```python
from build123d import *

# Parameters (mm, degrees)
SKETCH2_W           = 38.1
SKETCH2_H           = 76.2
BOSS_EXTRUDE1_DEPTH = 9.525
SKETCH3_OUTSIDE_W   = 57.246
SKETCH3_OUTSIDE_H   = 95.346
SKETCH3_OUTSIDE_W_2 = 38.1
SKETCH3_OUTSIDE_H_2 = 76.2
SKETCH3_OUTSIDE_R   = 4.318
CUT_EXTRUDE2_DEPTH  = 12.7


with BuildPart() as part:
    # Sketch2 → Boss-Extrude1 (new body)
    with BuildSketch(Plane.XY):
        Rectangle(SKETCH2_W, SKETCH2_H)
    extrude(amount=BOSS_EXTRUDE1_DEPTH)

    # Sketch3 outside → Cut-Extrude2 (cut)
    # profile 1 of 2: a face of its own
    with BuildSketch(Plane.XY.offset(9.525)):
        Rectangle(SKETCH3_OUTSIDE_W, SKETCH3_OUTSIDE_H)
        Rectangle(SKETCH3_OUTSIDE_W_2, SKETCH3_OUTSIDE_H_2, mode=Mode.SUBTRACT)
    # profile 2 of 2: a face of its own
    with BuildSketch(Plane.XY.offset(9.525)):
        Circle(SKETCH3_OUTSIDE_R)
    extrude(amount=-CUT_EXTRUDE2_DEPTH, mode=Mode.SUBTRACT)


solid = part.part
```
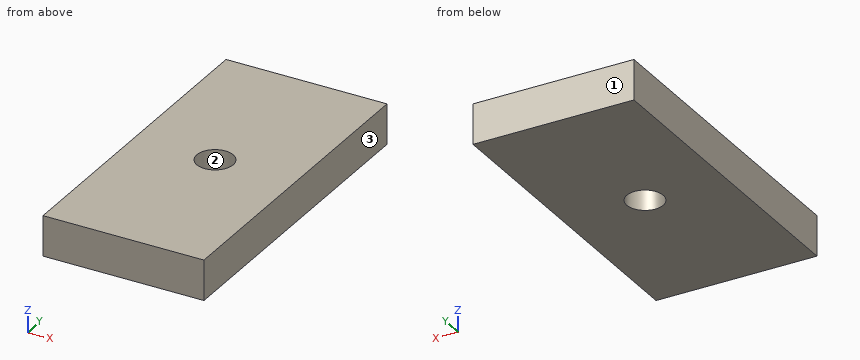
Build history of the part. All positions in model axes, mm. Face numbers are marked on the shaded views. Round coordinates to 2 decimals unless told otherwise and drop trailing zeros. Write each loop counter-clockwise with the first axis right and the second up, starting at its lowest first coordinate (ties: lowest second). Pieces come first, ordered by that corner, then holes. Notation, with made-up numbers: (39.25, 3.25) - (97.25, 3.25) arc R12 ccw to (97.25, 13.25) - close; hole circle Ø3 at (-37, -12). An arc over 180 degrees is marked (long way). Answer as CSV lines item,"result".
Q1. Pull direction Y, two halves, no side cores. Call the marked faces 1, 2 and 3: +Y half, -Y half, draft (parallel to the pull), parting line (faces both ways), or undercut.
Report:
face 1,"+Y half"
face 2,"undercut"
face 3,"draft"
Q2. Drill centre lines: probe 1 along Y at (x, z) = (0, 3.5); probe 2 along Y at (x, z) = (2, 7.75). Where is each one in solid material? Low to high. Write a range as [from, to].
Report:
probe 1,"y = [-38.1, -4.32], [4.32, 38.1]"
probe 2,"y = [-38.1, -3.83], [3.83, 38.1]"
Q3. Cut at B-B (z = 1). Write the cut outline in (x, y), and give its area (3 significant figures).
Report:
outline,"(-19.05, -38.1) - (19.05, -38.1) - (19.05, 38.1) - (-19.05, 38.1) - close; hole circle Ø8.64 at (0, 0)"
area,"2,840 mm^2"
Q4. Drop a flat-ended pin along its axis: pin 1 (5 mm diameter, centred on x = 0, y = 0, fed in from -Z). Give the stop position or say it passes through.
Report:
pin 1,"passes through"
Q5. Cut at A-A (y = 0). Write the cut outline in (x, z) (3 decimals), and give its area (3 significant figures).
Report:
outline,"(-19.05, 0) - (-4.318, 0) - (-4.318, 9.525) - (-19.05, 9.525) - close; (4.318, 0) - (19.05, 0) - (19.05, 9.525) - (4.318, 9.525) - close"
area,"281 mm^2"
Q6. Cut at C-C (x = 0). Write the cut outline in (y, z) (3 decimals).
Report:
outline,"(-38.1, 0) - (-4.318, 0) - (-4.318, 9.525) - (-38.1, 9.525) - close; (4.318, 0) - (38.1, 0) - (38.1, 9.525) - (4.318, 9.525) - close"
